from build123d import *

# Parameters (mm, degrees)
SKETCH_1_W               = 42
SKETCH_1_H               = 20
EXTRUDE_1_DEPTH          = 10
SKETCH_2_R               = 1.5
CUT_EXTRUDE_1_DEPTH      = 26.317977802
SKETCH_3_W               = 12
SKETCH_3_H               = 20
EXTRUDE_2_DEPTH          = 10
SKETCH_4_W               = 126.664391462
SKETCH_4_H               = 46.229783625
EXTRUDE_3_DEPTH          = 9.5
SKETCH_5_R               = 1.5
CUT_EXTRUDE_2_DEPTH      = 116.532726292
SKETCH_6_W               = 60
SKETCH_6_H               = 46.229783625
CUT_EXTRUDE_3_DEPTH      = 116.532726292
EXTRUDE_4_DEPTH          = 8
CUT_EXTRUDE_4_DEPTH      = 66.33057377
CUT_EXTRUDE_4_DEPTH_BACK = 66.33057377
RIB_1_REACH              = 87.25
SKETCH_10_WALL_W         = 201.667483308
SKETCH_10_WALL_H         = 8
CUT_EXTRUDE_5_DEPTH      = 62.626567883
EXTRUDE_5_DEPTH          = 8
FILLET_1_R               = 3
FILLET_2_R               = 4
FILLET_3_R               = 6


with BuildPart() as part:
    # 草图1 → 凸台-拉伸1 (new body)
    with BuildSketch(Plane(origin=(0, 0, 0), x_dir=(1, 0, 0), z_dir=(0, 1, 0))):
        Rectangle(SKETCH_1_W, SKETCH_1_H)
    extrude(amount=EXTRUDE_1_DEPTH)

    # 草图2 → 切除-拉伸1 (cut, through all)
    with BuildSketch(Plane(origin=(0, 10, 0), x_dir=(1, 0, 0), z_dir=(0, 1, 0))):
        with Locations(Location((-14, 5.5, 0), (0, 0, 270))):
            Circle(SKETCH_2_R)
        with Locations(Location((14, 5.5, 0), (0, 0, 90))):
            Circle(SKETCH_2_R)
        with Locations(Location((14, -5.5, 0), (0, 0, 270))):
            Circle(SKETCH_2_R)
        with Locations(Location((-14, -5.5, 0), (0, 0, 90))):
            Circle(SKETCH_2_R)
    extrude(amount=-CUT_EXTRUDE_1_DEPTH, mode=Mode.SUBTRACT)

    # 草图3 → 凸台-拉伸2 (add)
    with BuildSketch(Plane.XZ):
        with Locations((-27, 0)):
            Rectangle(SKETCH_3_W, SKETCH_3_H)
    extrude(amount=-EXTRUDE_2_DEPTH)

    # 草图4 → 凸台-拉伸3 (add)
    with BuildSketch(Plane.XY.offset(10)):
        with Locations((-42.332195731, -13.114891813)):
            Rectangle(SKETCH_4_W, SKETCH_4_H)
    extrude(amount=EXTRUDE_3_DEPTH)

    # 草图5 → 切除-拉伸2 (cut, through all)
    with BuildSketch(Plane.XY.offset(19.5)):
        with Locations((-34.435554727, -15.563062213)):
            Circle(SKETCH_5_R)
        with Locations((-6.689582963, -11.799945041)):
            Circle(SKETCH_5_R)
        with Locations((-5.211215503, -22.700148234)):
            Circle(SKETCH_5_R)
        with Locations((-32.957187267, -26.463265406)):
            Circle(SKETCH_5_R)
    extrude(amount=-CUT_EXTRUDE_2_DEPTH, mode=Mode.SUBTRACT)

    # 草图6 → 切除-拉伸3 (cut, through all)
    with BuildSketch(Plane.XY.offset(19.5)):
        with Locations((-75.664391462, -13.114891813)):
            Rectangle(SKETCH_6_W, SKETCH_6_H)
    extrude(amount=-CUT_EXTRUDE_3_DEPTH, mode=Mode.SUBTRACT)

    # 草图8 → 凸台-拉伸4 (add)
    with BuildSketch(Plane(origin=(21, 0, 0), x_dir=(0, 0, -1), z_dir=(1, 0, 0))):
        Polygon((-10, 0), (10, 0), (10, 10), (-19.5, 10), (-19.5, -36.229783625), (-10, -36.229783625), align=None)
    extrude(amount=EXTRUDE_4_DEPTH)

    # 草图9 → 切除-拉伸4 (cut, two sides: drawn at the far end of the back side and taken through both)
    with BuildSketch(Plane.XY.offset(19.5).offset(-CUT_EXTRUDE_4_DEPTH_BACK)):
        Polygon((29, -21.229783625), (-8.332195731, -36.229783625), (29, -36.229783625), align=None)
    extrude(amount=CUT_EXTRUDE_4_DEPTH + CUT_EXTRUDE_4_DEPTH_BACK, mode=Mode.SUBTRACT)

    # 草图10 wall → 筋1 (add, up to next)
    with BuildSketch(Plane(origin=(29, -10.614891812, 0), x_dir=(0, 0.727874330628, -0.685710550315), z_dir=(0, 0.685710550315, 0.727874330628)), mode=Mode.PRIVATE) as rib_1_sk1:
        with Locations((0, 4)):
            Rectangle(SKETCH_10_WALL_W, SKETCH_10_WALL_H)
    rib_1_tool1 = extrude(rib_1_sk1.sketch, amount=RIB_1_REACH, mode=Mode.PRIVATE) - part.part
    add(rib_1_tool1.solids().sort_by_distance((29, -10.614891812, 0))[0])

    # 草图12 → 切除-拉伸5 (cut, through all)
    with BuildSketch(Plane(origin=(0, 0, 10), x_dir=(-1, 0, 0), z_dir=(0, 0, -1))):
        Polygon((17.332195731, -36.229783625), (-21, -21.229783625), (-29, -21.229783625), (8.332195731, -36.229783625), align=None)
    extrude(amount=-CUT_EXTRUDE_5_DEPTH, mode=Mode.SUBTRACT)

    # 草图13 → 凸台-拉伸5 (add)
    with BuildSketch(Plane(origin=(-26.664391462, 0, 0), x_dir=(0, 0, -1), z_dir=(1, 0, 0))):
        Polygon((-10, -36.229783625), (10, 0), (-10, 0), align=None)
    extrude(amount=EXTRUDE_5_DEPTH)

    # 圆角1
    fillet_1_edges = [part.edges().sort_by_distance(p)[0] for p in [
        (21, 0, 0),
        (-26.664391462, 0, 0),
        (-18.664391462, 0, 0),
    ]]
    fillet(fillet_1_edges, radius=FILLET_1_R)

    # 圆角2
    fillet_2_edges = [part.edges().sort_by_distance(p)[0] for p in [
        (29, -21.229783625, 14.75),
    ]]
    fillet(fillet_2_edges, radius=FILLET_2_R)

    # 圆角3
    fillet_3_edges = [part.edges().sort_by_distance(p)[0] for p in [
        (-45.664391462, 10, 14.75),
        (-45.664391462, -36.229783625, 14.75),
    ]]
    fillet(fillet_3_edges, radius=FILLET_3_R)


solid = part.part
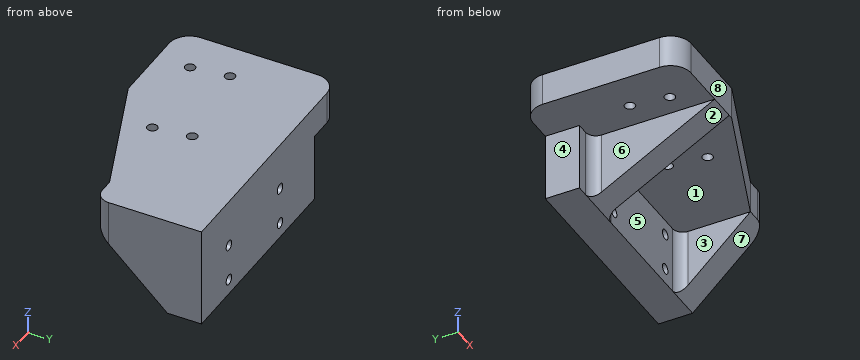
The model under review builds one solid part; all positions refer to its coordinate system, in mm. Face numbers are marked on the shaded views. A direction names the side the tool comes from. Round coordinates to 2 decimals unless told otherwise and drop trailing zeros. Order: outer loops, then holes, each group sorted by start corner. A loop starts at its lowest first (then second) coordinate and runs counter-clockwise, first axis right, second up. Notation, with made-up numbers: (-16.5, -31.5) -> (37.5, -31.5) arc R23 ccw to (37.5, -16.5) -> close; hole circle Ø1 at (59, 77.25). An arc over 180 degrees is marked (long way). Write item = value, one per line. Start each with the question number.
Item 1: For line 1 along X through (y, z) = (7.75, 5.5); line 2 along X through (y, z) = (-13, 9.75); line 3 along Z through (x, y) = (-31, -1.5), list the stretches that pass through material, from the lowest coordinate up.
Item 2: Consider section D-D on x = -23.5. Write out the cut boundary in (y, z).
Item 3: Consider section A-A on z = -5.75. Write out the cut boundary in (x, y), plus the area to 3 significant figures.
Item 4: For the marked faces 5, 6, 7 and 8, list the 3-axis set-ups (+Z, -Z, +X, -X, +Y, -Y) from which the entire face can be reached by the end or side of a thin tool; tool diameter is ignored.
Item 5: Mouldability with a two-part tool opening along X and no side actions: class the marked faces 1, 2, 3 and 4 as released by +X, released by -X, zero draft, split by the parting line, or undercut.
Item 6: Clearance check with flat-ended pins moving along their axes: pin 1 Ø2.5 at (x, z) = (-30.5, 0.5) entering from -Y; pin 2 Ø4.5 at (x, z) = (24, 12.5) entering from -Y; pin 3 Ø10 at (y, z) = (-6, -6) entering from -X; pin 4 Ø3 at (x, z) = (-18.5, 9) entering from -Y. State where each tip first meets the part, or that it passes through.
Item 7: Consider section C-C on y = -33. Write out the cut boundary in (x, z).
Item 8: Consider section B-B on x = -14. Write out the cut boundary in (y, z).
Conclusion:
q1.line_1 = -33 to -15.5, -12.5 to 12.5, 15.5 to 29
q1.line_2 = -26.66 to -18.66, 21 to 29
q1.line_3 = 10 to 19.5
q2.outline = (-36.23, 10) -> (0, -10) -> (10, -10) -> (10, 19.5) -> (-36.23, 19.5) -> close
q3.outline = (-33, 0) -> (-29.66, 0) arc R3 cw to (-26.66, -3) -> (-26.66, -7.7) -> (-18.66, -7.7) -> (-18.66, -3) arc R3 cw to (-15.66, 0) -> (-15.48, 0) -> (-15.48, 10) -> (-33, 10) -> close; (-12.52, 0) -> (12.52, 0) -> (12.52, 10) -> (-12.52, 10) -> close; (15.48, 0) -> (18, 0) arc R3 cw to (21, -3) -> (21, -4.51) -> (29, -4.51) -> (29, 10) -> (15.48, 10) -> close
q3.area = 664 mm2
q4.face_5 = -Z, -Y
q4.face_6 = -Z, -X, -Y
q4.face_7 = -Z, +X, -Y
q4.face_8 = +Z, -Z, +X, -X, -Y
q5.face_1 = undercut
q5.face_2 = zero draft
q5.face_3 = undercut
q5.face_4 = released by -X
q6.pin_1 = -0.03
q6.pin_2 = -21.23
q6.pin_3 = -27.43
q6.pin_4 = -36.23
q7.outline = (-44.99, 10) -> (-26.66, 10) -> (-26.66, 8.22) -> (-18.66, 8.22) -> (-18.66, 10) -> (-9.08, 10) -> (-9.08, 19.5) -> (-44.99, 19.5) -> close
q8.outline = (-34.93, 10) -> (0, 10) -> (0, 7) -> (10, 7) -> (10, 19.5) -> (-34.93, 19.5) -> close; (0, -10) -> (10, -10) -> (10, -7) -> (0, -7) -> close; (0, -4) -> (10, -4) -> (10, 4) -> (0, 4) -> close
